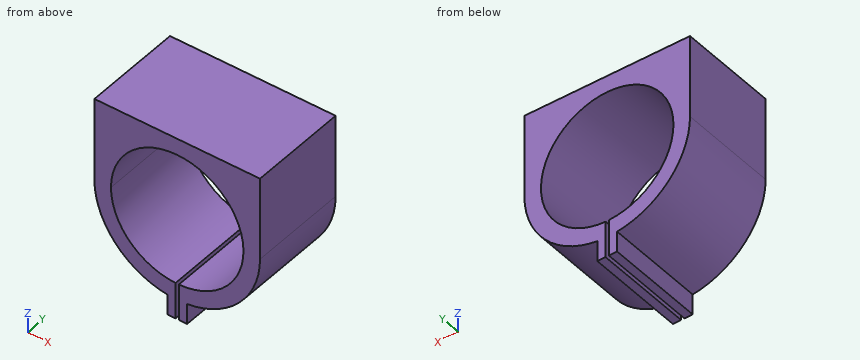
Autodesk Inventor part; units mm, degrees
ref_plane "YZ Plane" through (0, 0, 0) normal (1, 0, 0) x (0, 1, 0)
ref_plane "XZ Plane" through (0, 0, 0) normal (0, 1, 0) x (-1, 0, 0)
ref_plane "XY Plane" through (0, 0, 0) normal (0, 0, 1) x (1, 0, 0)
sketch "Sketch1" plane through (0, 0, 0) normal (0, 1, 0) x (-1, 0, 0)
  circle A0 centre (0, 0) radius 50
  circle A1 centre (0, 0) radius 40
  line L0 (50, 0) -> (-50, 0)
  line L1 (-50, 0) -> (-50, 50)
  line L2 (-50, 50) -> (50, 50)
  line L3 (50, 50) -> (50, 0)
  line L4 (6, -46) -> (-6, -46)
  line L5 (-6, -46) -> (-6, -62)
  line L6 (-6, -62) -> (6, -62)
  line L7 (6, -62) -> (6, -46)
  line L8 (1, -64) -> (-1, -64)
  line L9 (-1, -64) -> (-1, -35)
  line L10 (-1, -35) -> (1, -35)
  line L11 (1, -35) -> (1, -64)
  point P0 (1, -39.9875)
  point P1 (1, -62)
  point P2 (6, -49.6387)
  point P3 (-6, -49.6387)
  point P4 (-1, -62)
  point P5 (-1, -39.9875)
  dimension "d0" = 100
extrude "Extrusion1" add sketch "Sketch1" along normal blind 60 contours L0 A1 A0 | A0 L7 L4 L11 A1 L0 | A0 L2 L3 | A0 L1 L2 | L7 L6 L11 A0 | A0 L11 L4 L7 | L0 A1 L9 L4 L5 A0 | L5 L4 L9 A0 | A0 L9 L6 L5
properties part number "MotorClamp"
Work out the finished part from the listing and answer in its coordinate system (mm). Round coordinates to 2 decimals unless told otherwise and drop trailing zeros. Write each loop counter-clockwise with the first axis right and the second up, starting at its lowest first coordinate (ties: lowest second). Pieces come first, ordered by that corner, then holes. Notation, with made-up numbers: (-17, 76) -> (37, 76) arc R4 cw to (37, 83) -> close; hole circle Ø10 at (53, 86.5). An arc over 180 degrees is marked (long way). Answer as CSV lines item,"result". Start each with the question number.
(1) The part is cut by section C-C, the plane y = 45.5. Give the vertices of the cut face in (x, z), then the cut area to 3 significant figures.
(2) Each of these flat-tipped pins is pushed along its axis until it touches: pin 1 (3.5 mm diameter, centred on y = 44, z = -54, fed in from +X); pin 2 (24 mm diameter, centred on y = 23.5, z = -51.5, fed in from +X); pin 3 (10 mm diameter, centred on x = -16, y = 47.5, fed in from -Z) (3 decimals). Where does it stop, or does it pass through?
(3) The part is cut by section B-B, the plane x = 21. Give the vertices of the cut face in (y, z), then the cut area to 3 significant figures.
(4) The part is cut by section D-D, the plane x = -43. Give the vertices of the cut face in (y, z).
(5) The part is cut by section A-A, the plane z = -16.5. Give the vertices of the cut face in (x, y).
(6) Find the intervals of material crossed by probe 1 along X at (y, z) = (25, 0); probe 2 along Z at (x, y) = (0, 41.5); probe 3 along X at (y, z) = (21.5, -2.5), in increasing order.
Output values:
1,outline,"(-50, 0) arc R50 ccw to (-6, -49.64) -> (-6, -62) -> (-1, -62) -> (-1, -39.99) arc R40 cw (long way) to (1, -39.99) -> (1, -62) -> (6, -62) -> (6, -49.64) arc R50 ccw to (50, 0) -> (50, 50) -> (-50, 50) -> close"
1,area,"4,000 mm²"
2,pin 1,"stops at x = 6"
2,pin 2,"stops at x = 30.66"
2,pin 3,"stops at z = -48.775"
3,outline,"(0, -45.38) -> (60, -45.38) -> (60, -34.04) -> (0, -34.04) -> close; (0, 34.04) -> (60, 34.04) -> (60, 50) -> (0, 50) -> close"
3,area,"1,640 mm²"
4,outline,"(0, -25.51) -> (60, -25.51) -> (60, 50) -> (0, 50) -> close"
5,outline,"(-47.2, 0) -> (-36.44, 0) -> (-36.44, 60) -> (-47.2, 60) -> close; (36.44, 0) -> (47.2, 0) -> (47.2, 60) -> (36.44, 60) -> close"
6,probe 1,"x = -50 to -40, 40 to 50"
6,probe 2,"z = 40 to 50"
6,probe 3,"x = -49.94 to -39.92, 39.92 to 49.94"
